CAD build for the part. Positions are in the model's coordinates, mm. Coordinates: 2 decimals unless noted, no trailing zeros. Loops run counter-clockwise (first coordinate to the right, second up) from the corner with the lowest first, then second, coordinate; pieces in that order, holes last. Notation, with made-up numbers: (38.5, -13) - (70.5, -13) arc R22 cw to (70.5, 26) - close; hole circle Ø8 at (-2, 34). An arc over 180 degrees is marked (long way). Put each result on its own line as item: value.
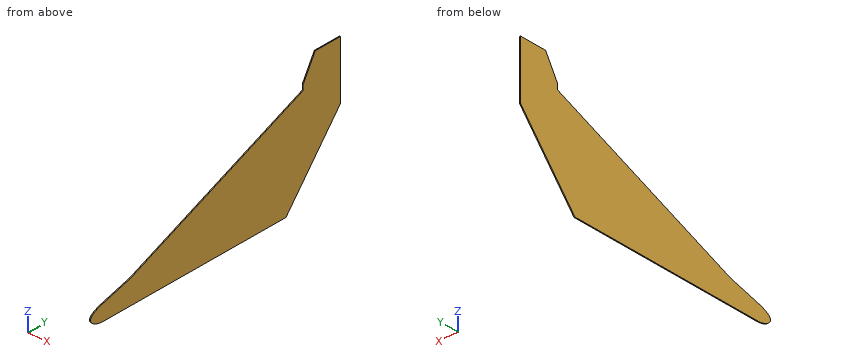
```python
from build123d import *

# Parameters (mm, degrees)
PAD_DEPTH    = 1.5
PAD002_DEPTH = 1.5


with BuildPart() as part:
    # Sketch → Pad (new body)
    with BuildSketch(Plane.YZ):
        with BuildLine():
            Line((130.835557, 163.892767), (34.582098, 103.74693))
            Line((34.582098, 103.74693), (34.582098, 95.464721))
            Line((34.582098, 95.464721), (-226.199079, 25.588615))
            add(Edge.make_bspline(
                [(-225, 0), (-241.014422, -1.461855), (-270.021739, 13.743032), (-226.199079, 25.588615)],
                knots=[0, 0, 0, 0, 1, 1, 1, 1], degree=3))
            Line((-225, 0), (100, 0))
            Line((100, 0), (197.335557, 116))
            Line((197.335557, 116), (197.335557, 210))
            Line((197.335557, 210), (152.335557, 210))
            Line((152.335557, 210), (130.835557, 172.760908))
            Line((130.835557, 172.760908), (130.835557, 163.892767))
        make_face()
    extrude(amount=PAD_DEPTH)

    # CopySketch003 → Pad002 (join)
    with BuildSketch(Plane.YZ):
        with BuildLine():
            Line((130.835557, 163.989908), (-177.902788, 38.529567))
            Line((-177.902788, 38.529567), (-226.199079, 25.588615))
            add(Edge.make_bspline(
                [(-225, 0), (-241.014422, -1.461855), (-270.021739, 13.743032), (-226.199079, 25.588615)],
                knots=[0, 0, 0, 0, 1, 1, 1, 1], degree=3))
            Line((-225, 0), (100, 0))
            Line((100, 0), (197.335557, 116))
            Line((197.335557, 116), (197.335557, 210))
            Line((197.335557, 210), (152.335557, 210))
            Line((152.335557, 210), (130.835557, 172.760908))
            Line((130.835557, 172.760908), (130.835557, 163.989908))
        make_face()
    extrude(amount=PAD002_DEPTH)


solid = part.part
```
Q1. Slice it at A-A, the plane z = 194. Give the cut face in (x, y), then the cut area to 3 significant figures.
Determined:
outline: (0, 143.1) - (1.5, 143.1) - (1.5, 197.34) - (0, 197.34) - close
area: 81.4 mm2
Q2. Wall check: L1, parallel to Z at x = 0.55, y = 151; L2, parallel to Y at x = 0.95, z = 20; L3, parallel to Z at x = 1.2, y = 118.5. Give the ranges that are in metal, low to high. Write a range as from..to.
Determined:
L1: 60.78..207.69
L2: -241.48..116.78
L3: 22.05..158.98
Q3. Slice it at B-B, the plane y = 19.5. Give the cut face in (x, z).
Determined:
outline: (0, 0) - (1.5, 0) - (1.5, 118.75) - (0, 118.75) - close
